from build123d import *

# Parameters (mm, degrees)
CROQUIS1_W                                 = 42.14
CROQUIS1_H                                 = 42.14
SALIENTE_EXTRUIR1_DEPTH                    = 48
CORTAR_EXTRUIR1_DEPTH                      = 53.151029
SIMETR_A3_AT_THE_SECOND_PLANE_COPY_1_DEPTH = 53.151029
CHAFL_N1_SIZE                              = 2.5
CROQUIS3_R                                 = 2.25
CORTAR_EXTRUIR2_DEPTH                      = 53.151029
SIMETR_A4_AT_THE_SECOND_PLANE_COPY_1_SKE_R = 2.25
SIMETR_A4_AT_THE_SECOND_PLANE_COPY_1_DEPTH = 53.151029
CROQUIS4_R                                 = 16.55
SALIENTE_EXTRUIR2_DEPTH                    = 2.5
CROQUIS6_R                                 = 2.58
SALIENTE_EXTRUIR4_DEPTH                    = 2
SALIENTE_EXTRUIR5_DEPTH                    = 18
SALIENTE_EXTRUIR3_DEPTH                    = 20
CHAFL_N2_SIZE                              = 2.5


with BuildPart() as part:
    # Croquis1 → Saliente-Extruir1 (new body)
    with BuildSketch(Plane(origin=(0, 0, 0), x_dir=(1, 0, 0), z_dir=(0, 1, 0))):
        Rectangle(CROQUIS1_W, CROQUIS1_H)
    extrude(amount=SALIENTE_EXTRUIR1_DEPTH)

    # Croquis2 → Cortar-Extruir1 (cut, through all)
    with BuildSketch(Plane(origin=(0, 42.8, 0), x_dir=(1, 0, 0), z_dir=(0, 1, 0))):
        with BuildLine():
            Line((-21.07, 12.72), (-16.895, 12.72))
            ThreePointArc((-16.895, 12.72), (-13.942829, 13.942829), (-12.72, 16.895))
            Line((-12.72, 16.895), (-12.72, 21.07))
            Line((-12.72, 21.07), (-21.07, 21.07))
            Line((-21.07, 21.07), (-21.07, 12.72))
        make_face()
    cortar_extruir1 = extrude(amount=-CORTAR_EXTRUIR1_DEPTH, mode=Mode.SUBTRACT)

    # Simetría3: Cortar-Extruir1 across plane
    add(cortar_extruir1.mirror(Plane(origin=(0, 0, 0), x_dir=(0, 0, 1), z_dir=(1, 0, 0))), mode=Mode.SUBTRACT)

    # Simetría3 at the second plane: Cortar-Extruir1 across plane
    add(cortar_extruir1.mirror(Plane.XY), mode=Mode.SUBTRACT)

    # Simetría3 at the second plane copy 1 ske → Simetría3 at the second plane copy 1 (cut, through all)
    with BuildSketch(Plane(origin=(0, 42.8, 0), x_dir=(-1, 0, 0), z_dir=(0, 1, 0))):
        with BuildLine():
            Line((-21.07, 12.72), (-16.895, 12.72))
            ThreePointArc((-16.895, 12.72), (-13.942829, 13.942829), (-12.72, 16.895))
            Line((-12.72, 16.895), (-12.72, 21.07))
            Line((-12.72, 21.07), (-21.07, 21.07))
            Line((-21.07, 21.07), (-21.07, 12.72))
        make_face()
    extrude(amount=-SIMETR_A3_AT_THE_SECOND_PLANE_COPY_1_DEPTH, mode=Mode.SUBTRACT)

    # Chaflán1
    chafl_n1_edges = [part.edges().sort_by_distance(p)[0] for p in [
        (-21.07, 21.4, -12.72),
        (-12.72, 21.4, -21.07),
        (-21.07, 21.4, 12.72),
        (-12.72, 21.4, 21.07),
        (21.07, 21.4, -12.72),
        (12.72, 21.4, -21.07),
        (21.07, 21.4, 12.72),
        (12.72, 21.4, 21.07),
    ]]
    chamfer(chafl_n1_edges, length=CHAFL_N1_SIZE)

    # Croquis3 → Cortar-Extruir2 (cut, through all)
    with BuildSketch(Plane.XZ.offset(-42.8)):
        with Locations(Location((16.895, -16.895, 0), (0, 0, 270))):
            Circle(CROQUIS3_R)
    cortar_extruir2 = extrude(amount=-CORTAR_EXTRUIR2_DEPTH, mode=Mode.SUBTRACT)

    # Simetría4: Cortar-Extruir2 across plane
    add(cortar_extruir2.mirror(Plane(origin=(0, 0, 0), x_dir=(0, 0, 1), z_dir=(1, 0, 0))), mode=Mode.SUBTRACT)

    # Simetría4 at the second plane: Cortar-Extruir2 across plane
    add(cortar_extruir2.mirror(Plane.XY), mode=Mode.SUBTRACT)

    # Simetría4 at the second plane copy 1 ske → Simetría4 at the second plane copy 1 (cut, through all)
    with BuildSketch(Plane(origin=(0, 42.8, 0), x_dir=(-1, 0, 0), z_dir=(0, -1, 0))):
        with Locations(Location((16.895, -16.895, 0), (0, 0, 270))):
            Circle(SIMETR_A4_AT_THE_SECOND_PLANE_COPY_1_SKE_R)
    extrude(amount=-SIMETR_A4_AT_THE_SECOND_PLANE_COPY_1_DEPTH, mode=Mode.SUBTRACT)

    # Croquis4 → Saliente-Extruir2 (add)
    with BuildSketch(Plane(origin=(0, 48, 0), x_dir=(1, 0, 0), z_dir=(0, 1, 0))):
        with Locations(Location((0, 0, 0), (0, 0, 270))):
            Circle(CROQUIS4_R)
    extrude(amount=SALIENTE_EXTRUIR2_DEPTH)

    # Croquis6 → Saliente-Extruir4 (add)
    with BuildSketch(Plane(origin=(0, 50.5, 0), x_dir=(1, 0, 0), z_dir=(0, 1, 0))):
        with Locations(Location((0, 0, 0), (0, 0, 270))):
            Circle(CROQUIS6_R)
    extrude(amount=SALIENTE_EXTRUIR4_DEPTH)

    # Croquis7 → Saliente-Extruir5 (add)
    with BuildSketch(Plane(origin=(0, 52.5, 0), x_dir=(1, 0, 0), z_dir=(0, 1, 0))):
        with BuildLine():
            Line((-1.379855, 2.18), (1.379855, 2.18))
            ThreePointArc((1.379855, 2.18), (0, -2.58), (-1.379855, 2.18))
        make_face()
    extrude(amount=SALIENTE_EXTRUIR5_DEPTH)

    # Croquis5 → Saliente-Extruir3 (add)
    with BuildSketch(Plane(origin=(0, 50.5, 0), x_dir=(1, 0, 0), z_dir=(0, 1, 0))):
        with BuildLine():
            Line((-1.379855, 2.18), (1.379855, 2.18))
            ThreePointArc((1.379855, 2.18), (0, -2.58), (-1.379855, 2.18))
        make_face()
    extrude(amount=SALIENTE_EXTRUIR3_DEPTH)

    # Chaflán2
    chafl_n2_edges = [part.edges().sort_by_distance(p)[0] for p in [
        (-21.07, 45.4, -21.07),
        (21.07, 45.4, -21.07),
        (21.07, 45.4, 21.07),
        (-21.07, 45.4, 21.07),
    ]]
    chamfer(chafl_n2_edges, length=CHAFL_N2_SIZE)


solid = part.part
Check sheet for the modelled part. Datum: model origin and axes. Units: mm. A direction names the side the tool comes from. Round coordinates to 2 decimals unless told otherwise and drop trailing zeros. Loops run counter-clockwise (first coordinate to the right, second up) from the corner with the lowest first, then second, coordinate; pieces in that order, holes last.
1. Mould release check, pull along X, two halves, no side actions. Record for faces 4 (the flat face through (15.7, 42.8, -14.5)), 5 (the cylindrical face through (-14.7, 45.4, -16.4)), 6 (the flat face through (-11.49, 21.7, 19.8)), 7 (the flat face through (19.8, 45.36, 19.84)): released by +X, released by -X, zero draft, split by the parting line, or undercut.
2. Sectioned sample at C-C on x = 0. Record the boundary of the cut face in (y, z), and give its area (3 significant figures).
3. Gauge pin test, flat ends, axial feed: pin 1 Ø0.8 at (y, z) = (15, 17.5) entering from -X; pin 2 Ø0.8 at (x, y) = (0.5, 60.5) entering from -Z; pin 3 Ø4 at (x, z) = (-16.5, -10) entering from +Y; pin 4 Ø4 at (x, z) = (16.895, 16.895) entering from +Y. Record the tip position at first contact, or that the pin passes through.
4. Set-up check for faces 1 (the flat face through (15.7, 42.8, 14.5)), 2 (the flat face through (18, 22, -12.72)), 3 (the cylindrical face through (4.971, 49.232, 15.786)): record each of +Z, -Z, +X, -X, +Y, -Y from which the full face is reachable in a straight line by a thin tool's end or side.
5. Sectioned sample at D-D on x = -8. Record the boundary of the cut face in (y, z).
6. Sectioned sample at B-B on y = 45. Record the boundary of the cut face in (x, z) (3 decimals).
7. Scan lines: probe 1 along Y at (x, z) = (5.5, 3.5); probe 2 along Y at (x, z) = (-0.5, -17.5); probe 3 along X at (y, z) = (33, 16.5). Record each from-to range of solid material in increasing order.
8. Sectioned sample at A-A on z = 0. Record the boundary of the cut face in (x, y).
Recorded:
1. face 4: zero draft
1. face 5: undercut
1. face 6: released by -X
1. face 7: released by +X
2. outline: (0, -21.07) - (48, -21.07) - (48, -16.55) - (50.5, -16.55) - (50.5, -2.58) - (52.5, -2.58) - (52.5, -2.18) - (70.5, -2.18) - (70.5, 2.58) - (50.5, 2.58) - (50.5, 16.55) - (48, 16.55) - (48, 21.07) - (0, 21.07) - close
2. area: 2,200 mm2
3. pin 1: stops at x = -12.72
3. pin 2: stops at z = -2.18
3. pin 3: stops at y = 48
3. pin 4: passes through
4. face 1: +Z, +X, -Y
4. face 2: -Z, +X, -Y
4. face 3: +Y
5. outline: (0, -21.07) - (48, -21.07) - (48, -14.49) - (50.5, -14.49) - (50.5, 14.49) - (48, 14.49) - (48, 21.07) - (0, 21.07) - close
6. outline: (-21.07, -18.57) - (-18.57, -21.07) - (18.57, -21.07) - (21.07, -18.57) - (21.07, 18.57) - (18.57, 21.07) - (-18.57, 21.07) - (-21.07, 18.57) - close; hole circle Ø4.5 at (-16.895, -16.895); hole circle Ø4.5 at (-16.895, 16.895); hole circle Ø4.5 at (16.895, -16.895); hole circle Ø4.5 at (16.895, 16.895)
7. probe 1: y = 0 to 50.5
7. probe 2: y = 0 to 48
7. probe 3: x = -12.74 to 12.74
8. outline: (-21.07, 0) - (21.07, 0) - (21.07, 48) - (16.55, 48) - (16.55, 50.5) - (2.58, 50.5) - (2.58, 70.5) - (-2.58, 70.5) - (-2.58, 50.5) - (-16.55, 50.5) - (-16.55, 48) - (-21.07, 48) - close
